Geometry: see drawing. Coordinates: mm, zero at the bounding-box minimum. A direction names the side the tool comes from. Give positions to 0.01 mm unless a question says otherwise; leave off trailing zeros. Loops run counter-clockwise (first coordinate to the right, second up) from the corner with the lowest first, then second, coordinate; pieces in that order, holes last. Notation, with made-up numbers: M 55.25,-10 L 66.25,-10 A11 ccw 66.25,0 Z; hole C 85.5,44.25 d10. An arc over 180 degrees is marked long. Put each result on its own line as item: value.
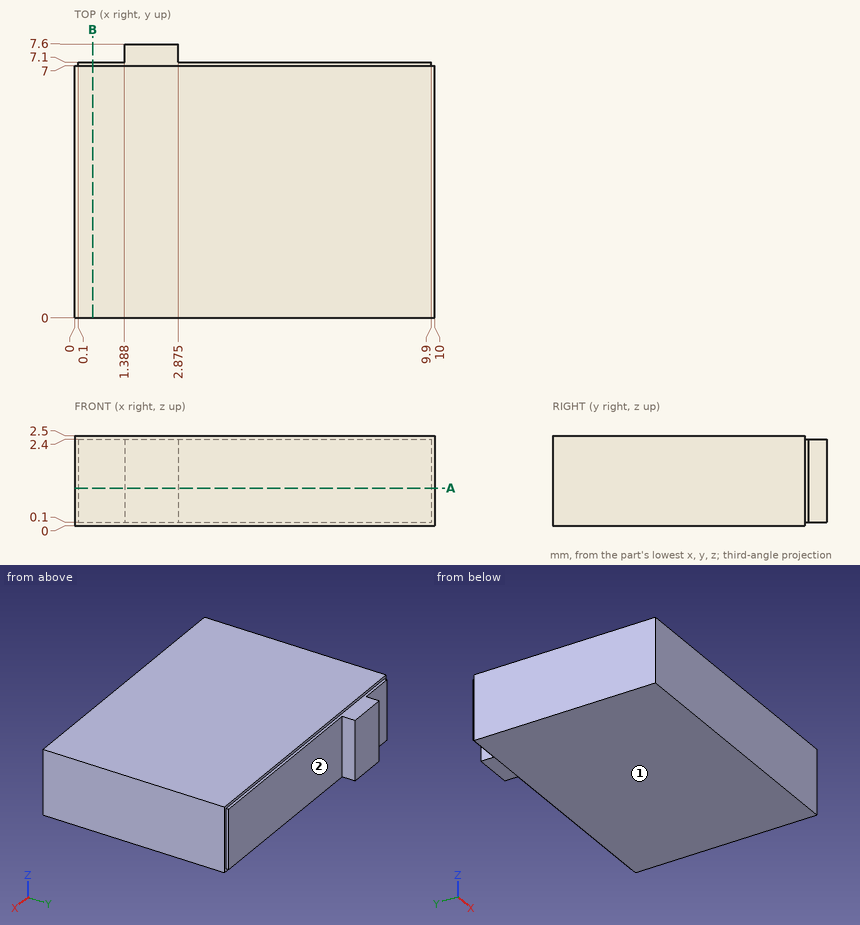
Item 1: Pin query (flat end, axial travel): pin 1 Ø1 at (x, z) = (4.5, 2) entering from +Y. Return the tip coordinate at first contact, or that it passes through.
Output values:
pin 1: y = 7.1
Item 2: Set-up query: the marked faces 1 and 2. Return all of +Z, -Z, +X, -X, +Y, -Y with unobstructed straight access to the full face (end or side cutting, diameter ignored); none if empty.
Output values:
face 1: -Z, +X, -X, +Y, -Y
face 2: +Z, -Z, +X, +Y
Item 3: Line query: probe 1 along Y at (x, z) = (6, 0.8); probe 2 along Y at (x, z) = (1.5, 2.45); probe 3 along X at (y, z) = (7.25, 0.8) (3 decimals). Output: solid intervals per line, ascending. Write a range as [from, to].
Output values:
probe 1: [0, 7.1]
probe 2: [0, 7]
probe 3: [1.388, 2.875]
Item 4: Section B-B on x = 0.5. Output: boundary loops of the cut face in (y, z).
Output values:
outline: M 0,0 L 7,0 L 7,0.1 L 7.1,0.1 L 7.1,2.4 L 7,2.4 L 7,2.5 L 0,2.5 Z
Item 5: Section A-A on z = 1.05. Output: boundary loops of the cut face in (x, y) (3 decimals), then the cut area to 3 significant figures.
Output values:
outline: M 0,0 L 10,0 L 10,7 L 9.9,7 L 9.9,7.1 L 2.875,7.1 L 2.875,7.6 L 1.388,7.6 L 1.388,7.1 L 0.1,7.1 L 0.1,7 L 0,7 Z
area: 71.7 mm²
